Autodesk Inventor part; units mm, degrees
ref_plane "YZ Plane" through (0, 0, 0) normal (1, 0, 0) x (0, 1, 0)
ref_plane "XZ Plane" through (0, 0, 0) normal (0, 1, 0) x (-1, 0, 0)
ref_plane "XY Plane" through (0, 0, 0) normal (0, 0, 1) x (1, 0, 0)
sketch "Sketch1" plane through (0, 0, 0) normal (1, 0, 0) x (0, 1, 0)
  line L0 (0, 0) -> (-32.9956, 19.05)
  line L1 (-32.9956, 19.05) -> (-28.5506, 26.749)
  line L2 (-28.5506, 26.749) -> (-6.35, 13.9315)
  line L3 (-6.35, 13.9315) -> (0, 13.9315)
  line L4 (0, 13.9315) -> (0, 10.8835)
  line L5 (0, 10.8835) -> (19.05, 10.8835)
  line L6 (19.05, 10.8835) -> (19.05, 6.9336)
  line L7 (19.05, 6.9336) -> (0, 0)
  dimension "d0" = 38.1
  dimension "d1" = 8.89
  dimension "d2" = 30
  dimension "d3" = 19.05
  dimension "d5" = 3.048
  dimension "d6" = 20
  dimension "d7" = 6.35
extrude "MAIN BODY" add sketch "Sketch1" along normal blind 50.8
sketch "Sketch2" plane through (0, 0, 10.8835) normal (0, 0, 1) x (1, 0, 0)
  line L0 (12.7, 9.398) -> (31.75, 9.398) construction
  line L1 (12.7, 5.588) -> (31.75, 5.588)
  line L2 (31.75, 13.208) -> (12.7, 13.208)
  arc A0 (12.7, 13.208) -> (12.7, 5.588) centre (12.7, 9.398) ccw
  arc A1 (31.75, 5.588) -> (31.75, 13.208) centre (31.75, 9.398) ccw
  line L3 (0, 19.05) -> (0, 0)
  line L4 (0, 19.05) -> (50.8, 19.05)
  line L5 (0, 0) -> (50.8, 0)
  point P0 (22.225, 9.398)
  dimension "d11" = 7.62
  dimension "d12" = 19.05
  dimension "d13" = 12.7
  dimension "d15" = 9.398
extrude "SLOT CUTOUT" cut sketch "Sketch2" against normal through all
sketch "Sketch3" plane through (0, -28.5506, 26.749) normal (0, 0.5, 0.8660254) x (1, 0, 0)
  circle A0 centre (19.05, 12.935) radius 6.35
  line L0 (38.1, 25.635) -> (50.8, 25.635)
  line L1 (50.8, 25.635) -> (50.8, 0)
  line L2 (50.8, 0) -> (38.1, 0)
  line L3 (38.1, 0) -> (38.1, 25.635)
  line L4 (0, 25.635) -> (0, 0)
  line L5 (0, 25.635) -> (50.8, 25.635)
  line L6 (50.8, 25.635) -> (50.8, 0)
  line L7 (0, 0) -> (50.8, 0)
  point P0 (0, 38.1)
  dimension "d18" = 12.7
  dimension "d19" = 19.05
  dimension "d20" = 12.7
  dimension "d21" = 38.1
extrude "CIRC AND RECT CUTOUT" cut sketch "Sketch3" against normal through all contours A0 | L0 L1 L2 L3
fillet ".25 filliets" radius 6.35 5 edges at (50.8, 19.05, 8.9085) (0, 19.05, 8.9085) (38.1, -8.5725, 10.082) (38.1, -30.7731, 22.8995) (0, -30.7731, 22.8995)
properties part number "ANS9-2-BK" material "Polypropylene"
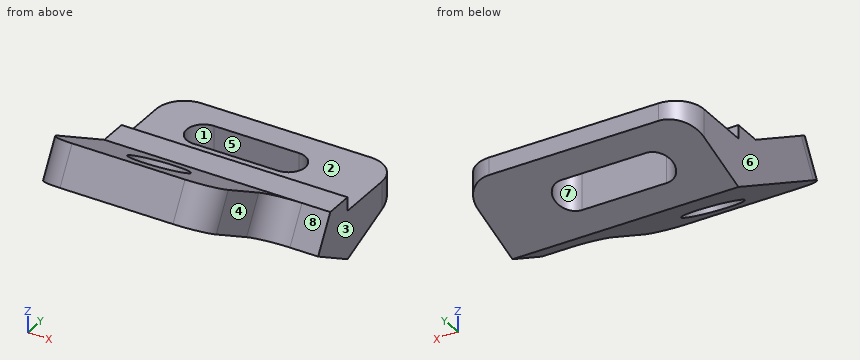
Build history of the part. All positions in model axes, mm. Face numbers are marked on the shaded views. A direction names the side the tool comes from. Coordinates: 2 decimals unless noted, no trailing zeros. Write each loop counter-clockwise with the first axis right and the second up, starting at its lowest first coordinate (ties: lowest second). Pieces come first, ordered by that corner, then holes. Notation, with made-up numbers: (-8, 46) -> (41, 46) arc R20 cw to (41, 73) -> close; hole circle Ø10 at (2.5, 84.25). An arc over 180 degrees is marked (long way). Use CSV: the item, a comma, the result in double quotes. Start each with the question number.
Q1. Cut at A-A, the plane x = 27. List the corners of the cut face in (y, z), then the cut area to 3 significant figures.
Q2. 3-axis set-ups, long thin cutter, end or side, ignore diameter. For the marked faces 1, 2, 3 and 4: which of +Z, -Z, +X, -X, +Y, -Y reach the whole face in a straight line?
Q3. Drill centre lines: probe 1 along Y at (x, z) = (4, 9.5); probe 2 along Y at (x, z) = (34.5, 8.5); probe 3 along Z at (x, y) = (39.5, -8). Where is each one in solid material? Low to high.
Q4. Cut at D-D, the plane x = 20.5. List the corners of the cut face in (y, z).
Q5. Cut at B-B, the plane x = 15. List the corners of the cut face in (y, z), then the cut area to 3 significant figures.
Q6. Cut at C-C, the plane x = 47. List the corners of the cut face in (y, z), then the cut area to 3 significant figures.
Q7. Pull direction Y, two halves, no side cores. Call the marked faces 5, 6, 7 and 8: released by +Y, released by -Y, zero draft, split by the parting line, or undercut.
Q8. Flat gauge pins, fed straight in: pin 1 Ø1.9 at (x, y) = (34, -4.5) entering from +Z; pin 2 Ø1 at (x, y) = (30, -27) entering from -Z; pin 3 Ø1.5 at (x, y) = (40, 12) entering from +Z. Where does each tip first touch, or does it go through?
Checked values:
1,outline,"(-33, 19.05) -> (0, 0) -> (5.59, 2.03) -> (5.59, 10.88) -> (0, 10.88) -> (0, 13.93) -> (-6.35, 13.93) -> (-28.55, 26.75) -> close; (13.21, 4.81) -> (19.05, 6.93) -> (19.05, 10.88) -> (13.21, 10.88) -> close"
1,area,"412 mm²"
2,face 1,"+Z, -Z"
2,face 2,"+Z, +X, -X, +Y"
2,face 3,"+Z, -Z, +X, +Y, -Y"
2,face 4,"+Z, +X, -Y"
3,probe 1,"y = -16.45 to 18.6"
3,probe 2,"y = -14.72 to 6.76, 12.03 to 19.05"
3,probe 3,"z = 4.62 to 14.88"
4,outline,"(-33, 19.05) -> (-27.15, 15.67) -> (-22.7, 23.37) -> (-28.55, 26.75) -> close; (-16.44, 9.49) -> (0, 0) -> (5.59, 2.03) -> (5.59, 10.88) -> (0, 10.88) -> (0, 13.93) -> (-6.35, 13.93) -> (-11.99, 17.19) -> close; (13.21, 4.81) -> (19.05, 6.93) -> (19.05, 10.88) -> (13.21, 10.88) -> close"
5,outline,"(-33, 19.05) -> (-26.03, 15.03) -> (-21.58, 22.73) -> (-28.55, 26.75) -> close; (-17.56, 10.14) -> (0, 0) -> (5.59, 2.03) -> (5.59, 10.88) -> (0, 10.88) -> (0, 13.93) -> (-6.35, 13.93) -> (-13.11, 17.84) -> close; (13.21, 4.81) -> (19.05, 6.93) -> (19.05, 10.88) -> (13.21, 10.88) -> close"
5,area,"325 mm²"
6,outline,"(-10.8, 6.23) -> (0, 0) -> (18.52, 6.74) -> (18.52, 10.88) -> (0, 10.88) -> (0, 13.93) -> (-6.35, 13.93) -> close"
6,area,"239 mm²"
7,face 5,"undercut"
7,face 6,"zero draft"
7,face 7,"undercut"
7,face 8,"released by -Y"
8,pin 1,"stops at z = 13.93"
8,pin 2,"stops at z = 15.3"
8,pin 3,"stops at z = 10.88"
